```python
from build123d import *

# Parameters (mm, degrees)
SKETCH1_W               = 180
SKETCH1_H               = 30
BOSS_EXTRUDE1_DEPTH     = 30
SKETCH2_R               = 11
CUT_EXTRUDE1_DEPTH      = 1
CUT_EXTRUDE1_DEPTH_BACK = 31
SKETCH3_W               = 23
SKETCH3_H               = 12
CUT_EXTRUDE2_DEPTH      = 1
CUT_EXTRUDE2_DEPTH_BACK = 181
SKETCH6_R               = 11
CUT_EXTRUDE5_DEPTH      = 1
CUT_EXTRUDE5_DEPTH_BACK = 31


with BuildPart() as part:
    # Sketch1 → Boss-Extrude1 (new body)
    with BuildSketch(Plane.XY):
        with Locations((35.284090909, 4.517045455)):
            Rectangle(SKETCH1_W, SKETCH1_H)
    extrude(amount=BOSS_EXTRUDE1_DEPTH)

    # Sketch2 → Cut-Extrude1 (cut, two sides)
    with BuildSketch(Plane(origin=(0, 19.517045455, 0), x_dir=(1, 0, 0), z_dir=(0, 1, 0))) as cut_extrude1_sk:
        with Locations((-40.715909091, -15)):
            Circle(SKETCH2_R)
    extrude(amount=CUT_EXTRUDE1_DEPTH, mode=Mode.SUBTRACT)
    extrude(cut_extrude1_sk.sketch, amount=-CUT_EXTRUDE1_DEPTH_BACK, mode=Mode.SUBTRACT)

    # Sketch3 → Cut-Extrude2 (cut, two sides)
    with BuildSketch(Plane.ZY.offset(54.715909091)) as cut_extrude2_sk:
        with Locations((15, 4.517045455)):
            Rectangle(SKETCH3_W, SKETCH3_H)
    extrude(amount=CUT_EXTRUDE2_DEPTH, mode=Mode.SUBTRACT)
    extrude(cut_extrude2_sk.sketch, amount=-CUT_EXTRUDE2_DEPTH_BACK, mode=Mode.SUBTRACT)

    # Sketch6 → Cut-Extrude5 (cut, two sides)
    with BuildSketch(Plane(origin=(0, 19.517045455, 0), x_dir=(1, 0, 0), z_dir=(0, 1, 0))) as cut_extrude5_sk:
        with Locations((111.284090909, -15)):
            Circle(SKETCH6_R)
    extrude(amount=CUT_EXTRUDE5_DEPTH, mode=Mode.SUBTRACT)
    extrude(cut_extrude5_sk.sketch, amount=-CUT_EXTRUDE5_DEPTH_BACK, mode=Mode.SUBTRACT)


solid = part.part
```
The model under review builds one solid part; all positions refer to its coordinate system, in mm. A direction names the side the tool comes from. Coordinates: 2 decimals unless noted, no trailing zeros. Order: outer loops, then holes, each group sorted by start corner. A loop starts at its lowest first (then second) coordinate and runs counter-clockwise, first axis right, second up. Notation, with made-up numbers: (-23.75, 49) -> (-17.75, 49) arc R17 cw to (-17.75, 68) -> close; hole circle Ø5 at (-28.75, 52.5). An arc over 180 degrees is marked (long way). Answer in a Markdown table with one row per item. Add a question column.
Item 1: We need section B-B on y = -3.5. Write out the cut boundary in (x, z), plus the area to 3 significant figures.
Item 2: To check wall thickness, follow probe 1 along X at (y, z) = (-8, 15); probe 2 along Y at (x, z) = (21.5, 24.25); probe 3 along X at (y, z) = (-5, 19.75). State the ranges of each line that lie inside material, in increasing order.
Item 3: We need section D-D on z = 6.5. Write out the cut boundary in (x, y).
Item 4: We need section C-C on x = 102.5. Write out the cut boundary in (y, z), plus the area to 3 significant figures.
Item 5: Machinability: for faces 1 (the flat face through (34, 10.517, 15)), 2 (the flat face through (34, 5, 30)), which of the approach directions +Z, -Z, +X, -X, +Y, -Y give a long, thin tool a straight path to every point of the face, cutting with its end or side? Answer none if there is none.
Item 6: Mouldability with a two-part tool opening along Z and no side actions: class faces 3 (the flat face through (125.284, -2, 15)), 4 (the flat face through (34, 4, 26.5)), 5 (the flat face through (34, 5, 0)) as +Z half, -Z half, draft (parallel to the pull), parting line (faces both ways), or undercut.
Item 7: We need section A-A on z = 15. Write out the cut boundary in (x, y).
Final values:
| question | item | result |
|---|---|---|
| 1 | outline | (-54.72, 0) -> (125.28, 0) -> (125.28, 30) -> (-54.72, 30) -> close; hole circle Ø22 at (-40.72, 15); hole circle Ø22 at (111.28, 15) |
| 1 | area | 4,640 mm2 |
| 2 | probe 1 | x = -54.72 to -51.72, -29.72 to 100.28, 122.28 to 125.28 |
| 2 | probe 2 | y = -10.48 to -1.48, 10.52 to 19.52 |
| 2 | probe 3 | x = -54.72 to -50.64, -30.79 to 101.36, 121.21 to 125.28 |
| 3 | outline | (-54.72, -10.48) -> (-47.7, -10.48) -> (-47.7, -1.48) -> (-54.72, -1.48) -> close; (-54.72, 10.52) -> (-47.7, 10.52) -> (-47.7, 19.52) -> (-54.72, 19.52) -> close; (-33.73, -10.48) -> (104.3, -10.48) -> (104.3, -1.48) -> (-33.73, -1.48) -> close; (-33.73, 10.52) -> (104.3, 10.52) -> (104.3, 19.52) -> (-33.73, 19.52) -> close; (118.27, -10.48) -> (125.28, -10.48) -> (125.28, -1.48) -> (118.27, -1.48) -> close; (118.27, 10.52) -> (125.28, 10.52) -> (125.28, 19.52) -> (118.27, 19.52) -> close |
| 4 | outline | (-10.48, 0) -> (19.52, 0) -> (19.52, 8.38) -> (10.52, 8.38) -> (10.52, 3.5) -> (-1.48, 3.5) -> (-1.48, 8.38) -> (-10.48, 8.38) -> close; (-10.48, 21.62) -> (-1.48, 21.62) -> (-1.48, 26.5) -> (10.52, 26.5) -> (10.52, 21.62) -> (19.52, 21.62) -> (19.52, 30) -> (-10.48, 30) -> close |
| 4 | area | 386 mm2 |
| 5 | face 1 | +X, -X |
| 5 | face 2 | +Z, +X, -X, +Y, -Y |
| 6 | face 3 | draft |
| 6 | face 4 | undercut |
| 6 | face 5 | -Z half |
| 7 | outline | (-54.72, -10.48) -> (-51.72, -10.48) -> (-51.72, -1.48) -> (-54.72, -1.48) -> close; (-54.72, 10.52) -> (-51.72, 10.52) -> (-51.72, 19.52) -> (-54.72, 19.52) -> close; (-29.72, -10.48) -> (100.28, -10.48) -> (100.28, -1.48) -> (-29.72, -1.48) -> close; (-29.72, 10.52) -> (100.28, 10.52) -> (100.28, 19.52) -> (-29.72, 19.52) -> close; (122.28, -10.48) -> (125.28, -10.48) -> (125.28, -1.48) -> (122.28, -1.48) -> close; (122.28, 10.52) -> (125.28, 10.52) -> (125.28, 19.52) -> (122.28, 19.52) -> close |
